The figure shows three views and two pictorial views of one solid part (mm, origin at its lowest corner). Answer the questions. A direction names the side the tool comes from. Coordinates: 2 decimals unless noted, no trailing zeros. Loops run counter-clockwise (first coordinate to the right, second up) from the corner with the lowest first, then second, coordinate; pieces in that order, holes last. Notation, with made-up numbers: M 64,86.25 L 110,86.25 A18 cw 110,116.25 Z; hole C 65.25,24 d4. An arc over 180 degrees is marked long. Return JSON: item names as keys, results as strings. Group by question number.
1. Section C-C (z = 45) is taken. Write down the section's boundary in (x, y), then the cut area to 3 significant figures.
2. Section B-B (y = 6.5) is taken. Write down the section's boundary in (x, z) (1 decimal).
3. Which of the six approach directions +Z, -Z, +X, -X, +Y, -Y give full straight-line access (tool end or side, diameter ignored) to the marked faces 1 and 2?
4. Section A-A (x = 44.5) is taken. Write down the section's boundary in (y, z) (1 decimal).
5. Straight lines are drawn through the part: L1, parallel to Y at x = 3.5, z = 7.5; L2, parallel to Z at x = 59.5, y = 13.5 (1 decimal). For each, find the intervals that lie inside material, in ascending order. Write a range as from..to.
6. Given P1, Ø20.5, axis at x = 31, y = 17.5, coming from the -Z side; P2, Ø23, axis at x = 29, z = 31.5, coming from the -Y side, each flat-ended and moving along its own axis, determine where each tip first touches the part or whether it passes through.
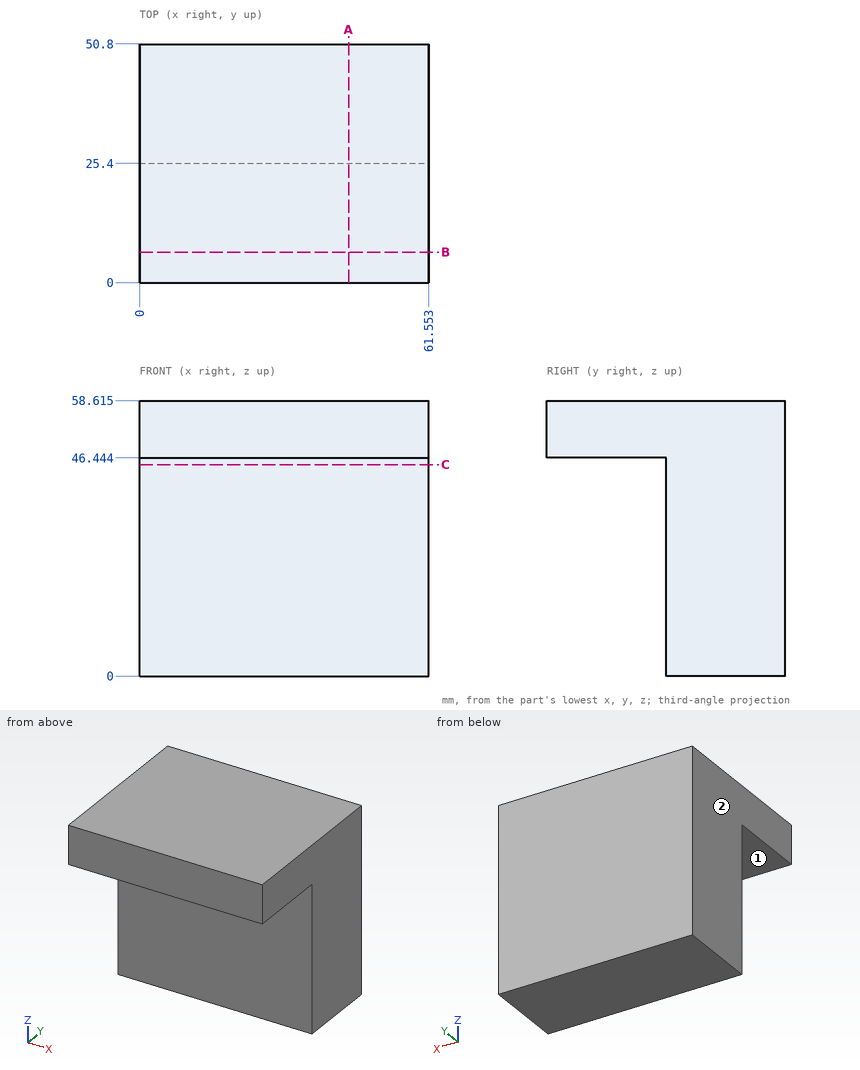
Worked out:
{
 "1": {"outline": "M 0,25.4 L 61.55,25.4 L 61.55,50.8 L 0,50.8 Z", "area": "1,560 mm^2"},
 "2": {"outline": "M 0,46.4 L 61.6,46.4 L 61.6,58.6 L 0,58.6 Z"},
 "3": {"face 1": "-Z, +X, -X, -Y", "face 2": "+Z, -Z, -X, +Y, -Y"},
 "4": {"outline": "M 0,46.4 L 25.4,46.4 L 25.4,0 L 50.8,0 L 50.8,58.6 L 0,58.6 Z"},
 "5": {"L1": "25.4..50.8", "L2": "46.4..58.6"},
 "6": {"P1": "z = 0", "P2": "y = 25.4"}
}
